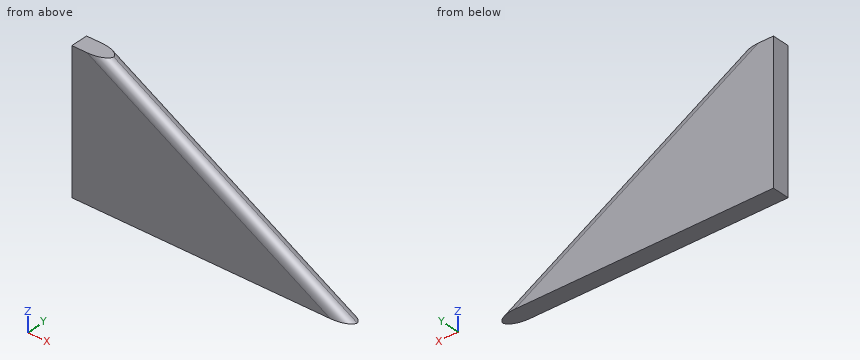
```python
from build123d import *

# Parameters (mm, degrees)
F1_DEPTH    = 3.175
F2_T1_DEPTH = 60.0853367017


# Not quite as in the source:
# - a fillet or chamfer that OpenCascade refuses, or shapes differently, is made with other operations: its cross-section is extruded or revolved along the edge and cut away or added


with BuildPart() as f1:
    # F0 (on Front) → F1 (new body)
    with BuildSketch(Plane.XZ):
        Polygon((0, 25.4), (0, 0), (50.8, 0), (6.35, 25.4), align=None)
    extrude(amount=F1_DEPTH)

    # F2: fillet of radius 1.778 on 2 edges, made by hand

    # F2_s2 → F2_t1 (cut)
    with BuildSketch(Plane(origin=(42.1547253821, 0, -24.0884145041), x_dir=(0, 1, 0), z_dir=(-0.8682431421, 0, 0.4961389384))):
        with BuildLine():
            ThreePointArc((-1.397, -25.2038580685), (-2.6542358569, -24.6830939255), (-3.175, -23.4258580685))
            Line((-3.175, -23.4258580685), (-3.175, -25.2038580685))
            Line((-3.175, -25.2038580685), (-1.397, -25.2038580685))
        make_face()
        with BuildLine():
            ThreePointArc((-1.778, -25.2038580685), (-0.5207641431, -24.6830939255), (0, -23.4258580685))
            Line((0, -23.4258580685), (0, -25.2038580685))
            Line((0, -25.2038580685), (-1.778, -25.2038580685))
        make_face()
    extrude(amount=F2_T1_DEPTH, mode=Mode.SUBTRACT)


solid = f1.part
```
Verification items for the finished model (mm, model axes). Coordinates: 2 decimals unless noted, no trailing zeros. Loops run counter-clockwise (first coordinate to the right, second up) from the corner with the lowest first, then second, coordinate; pieces in that order, holes last. Notation, with made-up numbers: (7.5, 43.25) -> (13.5, 43.25) arc R14 ccw to (13.5, 62.25) -> close; hole circle Ø10 at (53, 73.5). An arc over 180 degrees is marked (long way). Answer in a Markdown table with one row per item.
1) Section check A-A (y = -2.1). Record the cut outline in (x, z).
The answers:
| item | result |
|---|---|
| outline | (0, 0) -> (50.51, 0) -> (6.06, 25.4) -> (0, 25.4) -> close |
2) Depth check by flat-ended pin: P1, Ø1, axis at y = -1, z = 3, coming from the +X side. Enter the tip coordinate at first touch or a pass-through.
The answers:
| item | result |
|---|---|
| P1 | stops at x = 46.16 |
3) Scan lines: line 1 along Z through (x, y) = (24, -2.35); line 2 along Z through (x, y) = (22.5, -1.4); line 3 along X through (y, z) = (-1.9, 24.25). Record each from-to range of solid material in increasing order. Write a range as from..to.
The answers:
| item | result |
|---|---|
| line 1 | z = 0..15 |
| line 2 | z = 0..16.12 |
| line 3 | x = 0..8.22 |
